```python
from build123d import *

# Parameters (mm, degrees)
SKETCH1_R           = 4.5
SKETCH1_R_2         = 1
SKETCH1_R_3         = 12
SKETCH1_R_4         = 1.5
BOSS_EXTRUDE1_DEPTH = 3


with BuildPart() as part:
    # Sketch1 → Boss-Extrude1 (new body)
    with BuildSketch(Plane.XY):
        with BuildLine():
            ThreePointArc((-55.722139859, -57.402466232), (-15.796115106, -78.425013532), (29.155135021, -74.498175158))
            ThreePointArc((29.155135021, -74.498175158), (69.282032303, -40), (79.094879733, 12))
            ThreePointArc((79.094879733, 12), (40, 69.282032303), (-29.155135021, 74.498175158))
            ThreePointArc((-29.155135021, 74.498175158), (-78.425013532, 15.796115106), (-55.722139859, -57.402466232))
        make_face()
        with Locations((70, 0)):
            Circle(SKETCH1_R, mode=Mode.SUBTRACT)
        with Locations((77.425, 0)):
            Circle(SKETCH1_R_2, mode=Mode.SUBTRACT)
        with Locations((70, 7.425)):
            Circle(SKETCH1_R_2, mode=Mode.SUBTRACT)
        with Locations((62.575, 0)):
            Circle(SKETCH1_R_2, mode=Mode.SUBTRACT)
        with Locations((70, -7.425)):
            Circle(SKETCH1_R_2, mode=Mode.SUBTRACT)
        with Locations((35, -60.621778265)):
            Circle(SKETCH1_R, mode=Mode.SUBTRACT)
        with Locations((41.430238623, -56.909278265)):
            Circle(SKETCH1_R_2, mode=Mode.SUBTRACT)
        with Locations((38.7125, -67.052016888)):
            Circle(SKETCH1_R_2, mode=Mode.SUBTRACT)
        with Locations((28.569761377, -64.334278265)):
            Circle(SKETCH1_R_2, mode=Mode.SUBTRACT)
        with Locations((31.2875, -54.191539642)):
            Circle(SKETCH1_R_2, mode=Mode.SUBTRACT)
        with Locations((-35, -60.621778265)):
            Circle(SKETCH1_R, mode=Mode.SUBTRACT)
        with Locations((-28.569761377, -64.334278265)):
            Circle(SKETCH1_R_2, mode=Mode.SUBTRACT)
        with Locations((-38.7125, -67.052016888)):
            Circle(SKETCH1_R_2, mode=Mode.SUBTRACT)
        with Locations((-41.430238623, -56.909278265)):
            Circle(SKETCH1_R_2, mode=Mode.SUBTRACT)
        with Locations((-31.2875, -54.191539642)):
            Circle(SKETCH1_R_2, mode=Mode.SUBTRACT)
        with Locations((-70, 0)):
            Circle(SKETCH1_R, mode=Mode.SUBTRACT)
        with Locations((-70, -7.425)):
            Circle(SKETCH1_R_2, mode=Mode.SUBTRACT)
        with Locations((-77.425, 0)):
            Circle(SKETCH1_R_2, mode=Mode.SUBTRACT)
        with Locations((-70, 7.425)):
            Circle(SKETCH1_R_2, mode=Mode.SUBTRACT)
        with Locations((-62.575, 0)):
            Circle(SKETCH1_R_2, mode=Mode.SUBTRACT)
        with Locations((-35, 60.621778265)):
            Circle(SKETCH1_R, mode=Mode.SUBTRACT)
        with Locations((-41.430238623, 56.909278265)):
            Circle(SKETCH1_R_2, mode=Mode.SUBTRACT)
        with Locations((-38.7125, 67.052016888)):
            Circle(SKETCH1_R_2, mode=Mode.SUBTRACT)
        with Locations((-28.569761377, 64.334278265)):
            Circle(SKETCH1_R_2, mode=Mode.SUBTRACT)
        with Locations((-31.2875, 54.191539642)):
            Circle(SKETCH1_R_2, mode=Mode.SUBTRACT)
        with Locations((35, 60.621778265)):
            Circle(SKETCH1_R, mode=Mode.SUBTRACT)
        with Locations((28.569761377, 64.334278265)):
            Circle(SKETCH1_R_2, mode=Mode.SUBTRACT)
        with Locations((38.7125, 67.052016888)):
            Circle(SKETCH1_R_2, mode=Mode.SUBTRACT)
        with Locations((41.430238623, 56.909278265)):
            Circle(SKETCH1_R_2, mode=Mode.SUBTRACT)
        with Locations((31.2875, 54.191539642)):
            Circle(SKETCH1_R_2, mode=Mode.SUBTRACT)
        Circle(SKETCH1_R_3, mode=Mode.SUBTRACT)
        with Locations((0, 70)):
            Circle(SKETCH1_R_4, mode=Mode.SUBTRACT)
        with Locations((60.621778265, 35)):
            Circle(SKETCH1_R_4, mode=Mode.SUBTRACT)
        with Locations((60.621778265, -35)):
            Circle(SKETCH1_R_4, mode=Mode.SUBTRACT)
        with Locations((0, -70)):
            Circle(SKETCH1_R_4, mode=Mode.SUBTRACT)
        with Locations((-60.621778265, -35)):
            Circle(SKETCH1_R_4, mode=Mode.SUBTRACT)
        with Locations((-60.621778265, 35)):
            Circle(SKETCH1_R_4, mode=Mode.SUBTRACT)
        with BuildLine():
            Line((-36.545698507, 39.299006612), (-25.11473671, 19.5))
            ThreePointArc((-25.11473671, 19.5), (-25.11473671, 14.5), (-29.444863729, 12))
            Line((-29.444863729, 12), (-52.306787322, 12))
            ThreePointArc((-52.306787322, 12), (-56.351986497, 14.061230932), (-57.061949806, 18.545454545))
            ThreePointArc((-57.061949806, 18.545454545), (-51.961524227, 30), (-44.591809664, 40.144370849))
            ThreePointArc((-44.591809664, 40.144370849), (-40.353376444, 41.771636394), (-36.545698507, 39.299006612))
        make_face(mode=Mode.SUBTRACT)
        with BuildLine():
            Line((15.761088816, 51.299006612), (4.330127019, 31.5))
            ThreePointArc((4.330127019, 31.5), (0, 29), (-4.330127019, 31.5))
            Line((-4.330127019, 31.5), (-15.761088816, 51.299006612))
            ThreePointArc((-15.761088816, 51.299006612), (-15.998610053, 55.832867326), (-12.470140142, 58.689825394))
            ThreePointArc((-12.470140142, 58.689825394), (0, 60), (12.470140142, 58.689825394))
            ThreePointArc((12.470140142, 58.689825394), (15.998610053, 55.832867326), (15.761088816, 51.299006612))
        make_face(mode=Mode.SUBTRACT)
        with BuildLine():
            Line((36.545698507, 39.299006612), (25.11473671, 19.5))
            ThreePointArc((25.11473671, 19.5), (25.11473671, 14.5), (29.444863729, 12))
            Line((29.444863729, 12), (52.306787322, 12))
            ThreePointArc((52.306787322, 12), (56.351986497, 14.061230932), (57.061949806, 18.545454545))
            ThreePointArc((57.061949806, 18.545454545), (51.961524227, 30), (44.591809664, 40.144370849))
            ThreePointArc((44.591809664, 40.144370849), (40.353376444, 41.771636394), (36.545698507, 39.299006612))
        make_face(mode=Mode.SUBTRACT)
        with BuildLine():
            Line((52.306787322, -12), (29.444863729, -12))
            ThreePointArc((29.444863729, -12), (25.11473671, -14.5), (25.11473671, -19.5))
            Line((25.11473671, -19.5), (36.545698507, -39.299006612))
            ThreePointArc((36.545698507, -39.299006612), (40.353376444, -41.771636394), (44.591809664, -40.144370849))
            ThreePointArc((44.591809664, -40.144370849), (51.961524227, -30), (57.061949806, -18.545454545))
            ThreePointArc((57.061949806, -18.545454545), (56.351986497, -14.061230932), (52.306787322, -12))
        make_face(mode=Mode.SUBTRACT)
        with BuildLine():
            Line((15.761088816, -51.299006612), (4.330127019, -31.5))
            ThreePointArc((4.330127019, -31.5), (0, -29), (-4.330127019, -31.5))
            Line((-4.330127019, -31.5), (-15.761088816, -51.299006612))
            ThreePointArc((-15.761088816, -51.299006612), (-15.998610053, -55.832867326), (-12.470140142, -58.689825395))
            ThreePointArc((-12.470140142, -58.689825395), (0, -60), (12.470140142, -58.689825394))
            ThreePointArc((12.470140142, -58.689825394), (15.998610053, -55.832867326), (15.761088816, -51.299006612))
        make_face(mode=Mode.SUBTRACT)
        with BuildLine():
            Line((-36.545698507, -39.299006612), (-25.11473671, -19.5))
            ThreePointArc((-25.11473671, -19.5), (-25.11473671, -14.5), (-29.444863729, -12))
            Line((-29.444863729, -12), (-52.306787322, -12))
            ThreePointArc((-52.306787322, -12), (-56.351986497, -14.061230932), (-57.061949806, -18.545454545))
            ThreePointArc((-57.061949806, -18.545454545), (-51.961524227, -30), (-44.591809664, -40.144370849))
            ThreePointArc((-44.591809664, -40.144370849), (-40.353376444, -41.771636394), (-36.545698507, -39.299006612))
        make_face(mode=Mode.SUBTRACT)
    extrude(amount=BOSS_EXTRUDE1_DEPTH)


solid = part.part
```
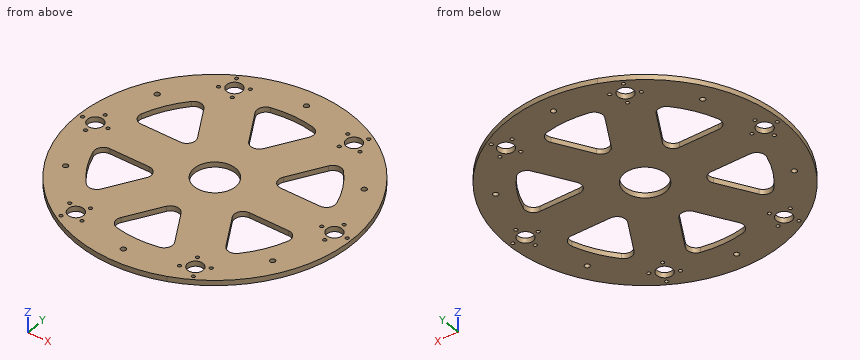
Verification items for the finished model (mm, model axes). Coordinates: 2 decimals unless noted, no trailing zeros. Loops run counter-clockwise (first coordinate to the right, second up) from the corner with the lowest first, then second, coordinate; pieces in that order, holes last. Notation, with made-up numbers: (86.5, -11) - (101.5, -11) arc R20 cw to (101.5, 8) - close; hole circle Ø10 at (-4, -10.5). An arc over 180 degrees is marked (long way). Answer as a JSON object with one key per item and string values.
(1) Cross-section at B-B, the plane x = 8.5. Record the boundary of the cut face in (y, z).
Response:
{"outline": "(-79.55, 0) - (-59.39, 0) - (-59.39, 3) - (-79.55, 3) - close; (-38.72, 0) - (-8.47, 0) - (-8.47, 3) - (-38.72, 3) - close; (8.47, 0) - (38.72, 0) - (38.72, 3) - (8.47, 3) - close; (59.39, 0) - (79.55, 0) - (79.55, 3) - (59.39, 3) - close"}
(2) Go/stop test with flat-tipped pins: pin 1 Ø1.2 at (x, y) = (-28.57, 64.33) entering from +Z; pin 2 Ø10 at (x, y) = (-39.5, -39) entering from +Z; pin 3 Ø1 at (x, z) = (-29, 1.5) entering from +Y; pin 4 Ø1.5 at (x, z) = (-36, 1) entering from +Y. Record where each tip stops, or that it passes through.
Response:
{"pin 1": "passes through", "pin 2": "stops at z = 3", "pin 3": "stops at y = 74.75", "pin 4": "stops at y = 71.82"}
(3) Scan lines: line 1 along Y through (x, z) = (25, 0.9); line 2 along X through (y, z) = (-36, 1.25); line 3 along Y through (x, z) = (2, 2.1) (3 decimals). Record each from-to range of solid material in increasing order.
Response:
{"line 1": "y = -75.99 to -19.29, -14.71 to 14.71, 19.29 to 75.99", "line 2": "x = -71.44 to -61.74, -59.5 to -48, -34.64 to -6.93, 6.93 to 34.64, 48 to 59.5, 61.74 to 71.44", "line 3": "y = -79.975 to -59.967, -29.417 to -11.832, 11.832 to 29.417, 59.967 to 79.975"}
(4) Cross-section at C-C, the plane y = -25. Record the boundary of the cut face in (x, z), then the cut area to 3 significant figures.
Response:
{"outline": "(-75.99, 0) - (-54.54, 0) - (-54.54, 3) - (-75.99, 3) - close; (-28.29, 0) - (28.29, 0) - (28.29, 3) - (-28.29, 3) - close; (54.54, 0) - (75.99, 0) - (75.99, 3) - (54.54, 3) - close", "area": "298 mm²"}
(5) Cross-section at D-D, the plane z = 1.55. Count the separate pieces of the cut face and the enclosed holes in it, then the cut area to 3 significant figures.
Response:
{"separate pieces": "1", "enclosed holes": "43", "area": "15,200 mm²"}
(6) Cross-section at A-A, the plane x = 47. Record the boundary of the cut face in (y, z).
Response:
{"outline": "(-64.74, 0) - (-37.3, 0) - (-37.3, 3) - (-64.74, 3) - close; (-12, 0) - (12, 0) - (12, 3) - (-12, 3) - close; (37.3, 0) - (64.74, 0) - (64.74, 3) - (37.3, 3) - close"}
